Verification items for the finished model (mm, model axes). Face numbers are marked on the shaded views. A direction names the side the tool comes from. Give positions to 0.01 mm unless a question says otherwise; leave off trailing zeros. Order: outer loops, then holes, each group sorted by start corner. A loop starts at its lowest first (then second) coordinate and runs counter-clockwise, first axis right, second up. Notation, with made-up numbers: (82, 5) - (119, 5) arc R20 ccw to (119, 21) - close; hole circle Ø2 at (-18, -24.75). An arc over 180 degrees is marked (long way). Answer as a JSON object with one key per item and string values. Group by question number.
(1) Section check D-D (z = 7.5). Record the boundary of the cut face in (x, y), then the cut area to 3 significant figures.
(2) Section check C-C (y = 3.7). Record the boundary of the cut face in (x, z).
(3) Access from +Z, -Z, +X, -X, +Y, -Y to the whole of each face (thin tool, end or side, straight path). Record for the marked faces 1 and 2.
(4) Depth check by flat-ended pin: pin 1 Ø3 at (y, z) = (2, 8) entering from +X; pin 2 Ø2 at (y, z) = (3.5, 26) entering from -X; pin 3 Ø0.8 at (x, y) = (7, 1) entering from +Z. Enter the tip coordinate at first touch or a pass-through.
(5) Section check B-B (x = 9). Record the boundary of the cut face in (y, z).
(6) Section check A-A (z = 24). Record the boundary of the cut face in (x, y).
(7) Thickness scan on line 1 (Y direction, x = 2.8, z = 7.5); line 2 (X direction, y = 0.6, z = 23.5); line 3 (X direction, y = 3.45, z = 44). Record the ranges inside material, lowest first.
(8) Mould release check, pull along X, two halves, no side actions. Record for the marked faces 3, 4, 5 and 6: +X half, -X half, draft (parallel to the pull), parting line (faces both ways), or undercut.
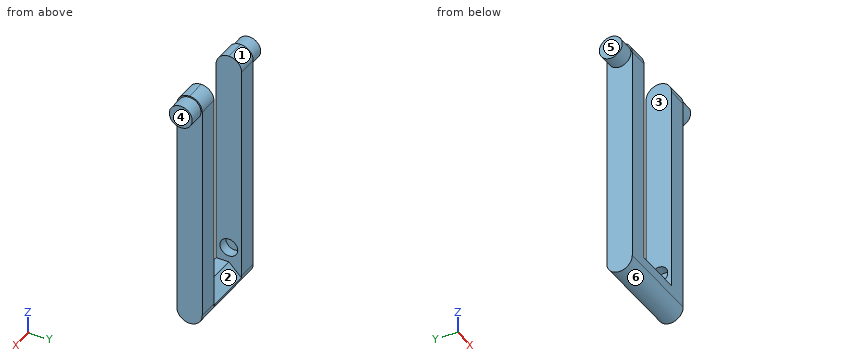
```python
from build123d import *

# Parameters (mm, degrees)
BOSS_EXTRUDE1_DEPTH     = 5
SKETCH2_R               = 2.25
BOSS_EXTRUDE2_DEPTH     = 3
FILLET3_R               = 2.5
BOSS_EXTRUDE3_START     = 3
SKETCH3_R               = 2.25
BOSS_EXTRUDE3_DEPTH     = 3
FILLET4_R               = 2.5
CHAMFER1_START          = 4.949747468
CHAMFER1_OUTLINE_W      = 9.5
CHAMFER1_OUTLINE_H      = 3.535533906
CHAMFER1_DEPTH          = 3.050252532
FILLET5_R               = 2.5
CUT_EXTRUDE1_DEPTH      = 11.5
CUT_EXTRUDE1_DEPTH_BACK = 2
SKETCH4_R               = 1.75


with BuildPart() as part:
    # Sketch1 → Boss-Extrude1 (new body)
    with BuildSketch(Plane(origin=(0, 0, 0), x_dir=(1, 0, 0), z_dir=(0, 1, 0))):
        Polygon((17.5, 0), (0, 0), (0, -47.5), (4, -47.5), (4, -4.5), (13.5, -4.5), (13.5, -47.5), (17.5, -47.5), align=None)
    extrude(amount=BOSS_EXTRUDE1_DEPTH)

    # Sketch2 → Boss-Extrude2 (add)
    with BuildSketch(Plane(origin=(17.5, 0, 0), x_dir=(0, 0, -1), z_dir=(1, 0, 0))):
        with Locations((-45, 2.5)):
            Circle(SKETCH2_R)
    extrude(amount=BOSS_EXTRUDE2_DEPTH)

    # Fillet3
    fillet3_edges = [part.edges().sort_by_distance(p)[0] for p in [
        (15.5, 0, 47.5),
        (15.5, 5, 47.5),
    ]]
    fillet(fillet3_edges, radius=FILLET3_R - 0.0001)  # a hair under: the kernel refuses the full size

    # Sketch3 → Boss-Extrude3 (add)
    with BuildSketch(Plane.ZY.offset(BOSS_EXTRUDE3_START)):
        with Locations(Location((45, 2.5, 0), (0, 0, 180))):
            Circle(SKETCH3_R)
    extrude(amount=-BOSS_EXTRUDE3_DEPTH)

    # Fillet4
    fillet4_edges = [part.edges().sort_by_distance(p)[0] for p in [
        (2, 0, 47.5),
        (2, 5, 47.5),
    ]]
    fillet(fillet4_edges, radius=FILLET4_R - 0.0001)  # a hair under: the kernel refuses the full size

    # Chamfer1: read off the stored shape, not the designer's step
    # Chamfer1 outline → Chamfer1 (cut)
    with BuildSketch(Plane(origin=(0, 0, 0), x_dir=(1, 0, 0), z_dir=(0, 0.7071067811865476, 0.7071067811865476)).offset(CHAMFER1_START)):
        with Locations((8.75, 0.353553391)):
            Rectangle(CHAMFER1_OUTLINE_W, CHAMFER1_OUTLINE_H)
    extrude(amount=CHAMFER1_DEPTH, mode=Mode.SUBTRACT)

    # Fillet5
    # the kernel refuses this fillet: 2.5 mm, written as the material it takes off along each edge
    with BuildSketch(Plane(origin=(23.75, 0, 0), x_dir=(0, 0, 1), z_dir=(-1, 0, 0))) as fillet5_piece_1:
        with BuildLine():
            CenterArc((FILLET5_R, FILLET5_R), FILLET5_R, 180, 90)
            Line((0, FILLET5_R), (0, 0))
            Line((0, 0), (FILLET5_R, 0))
        make_face()
    extrude(amount=30, mode=Mode.SUBTRACT)
    with BuildSketch(Plane(origin=(23.75, 5, 0), x_dir=(0, 0, 1), z_dir=(-1, 0, 0))) as fillet5_piece_2:
        with BuildLine():
            CenterArc((FILLET5_R, -FILLET5_R), FILLET5_R, 90, 90)
            Line((0, -FILLET5_R), (0, 0))
            Line((0, 0), (FILLET5_R, 0))
        make_face()
    extrude(amount=30, mode=Mode.SUBTRACT)

    # Sketch4 → Cut-Extrude1 (cut, two sides: drawn at the far end of the back side and taken through both)
    with BuildSketch(Plane.ZY.offset(-13.5).offset(-CUT_EXTRUDE1_DEPTH_BACK)):
        with Locations((7.5, 2.5)):
            Circle(SKETCH4_R)
    extrude(amount=CUT_EXTRUDE1_DEPTH + CUT_EXTRUDE1_DEPTH_BACK, mode=Mode.SUBTRACT)


solid = part.part
```
Solutions:
{
 "1": {"outline": "(0, 0) - (4, 0) - (4, 0.75) - (2, 0.75) - (2, 4.25) - (4, 4.25) - (4, 5) - (0, 5) - close; (13.5, 0) - (17.5, 0) - (17.5, 5) - (13.5, 5) - (13.5, 4.25) - (15.5, 4.25) - (15.5, 0.75) - (13.5, 0.75) - close", "area": "26.0 mm2"},
 "2": {"outline": "(-3, 43.1) - (0, 43.1) - (0, 0.31) - (17.5, 0.31) - (17.5, 43.1) - (20.5, 43.1) - (20.5, 46.9) - (17.5, 46.9) - (17.5, 47.19) - (13.5, 47.19) - (13.5, 8.77) - (15.5, 8.77) - (15.5, 6.23) - (13.5, 6.23) - (13.5, 3.3) - (4, 3.3) - (4, 6.23) - (2, 6.23) - (2, 8.77) - (4, 8.77) - (4, 47.19) - (0, 47.19) - (0, 46.9) - (-3, 46.9) - close"},
 "3": {"face 1": "+Z, +X, -X, +Y", "face 2": "+Z, +Y"},
 "4": {"pin 1": "stops at x = 17.5", "pin 2": "stops at x = 0", "pin 3": "stops at z = 4.5"},
 "5": {"outline": "(0, 2.5) arc R2.5 ccw to (4.96, 2.04) - (2.5, 4.5) - (0, 4.5) - close"},
 "6": {"outline": "(0, 0) - (4, 0) - (4, 5) - (0, 5) - close; (13.5, 0) - (17.5, 0) - (17.5, 5) - (13.5, 5) - close"},
 "7": {"line 1": "y = 0 to 0.75, 4.25 to 5", "line 2": "x = 0 to 4, 13.5 to 17.5", "line 3": "x = -3 to 4, 13.5 to 20.5"},
 "8": {"face 3": "undercut", "face 4": "+X half", "face 5": "-X half", "face 6": "draft"}
}
